from build123d import *

# Parameters (mm, degrees)
CROQUIS1_W              = 70
CROQUIS1_H              = 22
SALIENTE_EXTRUIR1_DEPTH = 18
CROQUIS2_R              = 2.5
SALIENTE_EXTRUIR2_DEPTH = 10
REDONDEO3_R             = 5
REDONDEO4_R             = 5


with BuildPart() as part:
    # Croquis1 → Saliente-Extruir1 (new body)
    with BuildSketch(Plane.XY):
        with Locations((35, 11)):
            Rectangle(CROQUIS1_W, CROQUIS1_H)
    extrude(amount=SALIENTE_EXTRUIR1_DEPTH)

    # Croquis2 → Saliente-Extruir2 (add)
    with BuildSketch(Plane.XY.offset(18)):
        with Locations(Location((59.5, 11, 0), (0, 0, 180))):
            Circle(CROQUIS2_R)
    extrude(amount=SALIENTE_EXTRUIR2_DEPTH)

    # Redondeo3
    redondeo3_edges = [part.edges().sort_by_distance(p)[0] for p in [
        (0, 22, 9),
    ]]
    fillet(redondeo3_edges, radius=REDONDEO3_R)

    # Redondeo4
    redondeo4_edges = [part.edges().sort_by_distance(p)[0] for p in [
        (0, 0, 9),
    ]]
    fillet(redondeo4_edges, radius=REDONDEO4_R)


solid = part.part
The model under review builds one solid part; all positions refer to its coordinate system, in mm. A direction names the side the tool comes from. Give positions to 0.01 mm unless a question says otherwise; leave off trailing zeros. Order: outer loops, then holes, each group sorted by start corner. A loop starts at its lowest first (then second) coordinate and runs counter-clockwise, first axis right, second up. Notation, with made-up numbers: (87, 46) -> (98, 46) arc R19 ccw to (98, 61) -> close; hole circle Ø11 at (47.5, 67.5). An arc over 180 degrees is marked (long way). Write item = value, one per line. Start each with the question number.
(1) Take a section at A-A (y = 11). Write out the cut boundary in (x, z).
(2) Take a section at B-B (x = 59.5). Write out the cut boundary in (y, z).
(3) For L1, parallel to Z at x = 28, y = 17; L2, parallel to X at y = 19.75, z = 6.5; L3, parallel to Y at x = 4, z = 8.75, list the stretches that pass through material, from the lowest coordinate up. Write a range as from..to.
(4) Tool access review of faces 1 (the flat face through (70, 11, 9)), 2 (the cylindrical face through (57.19, 11.96, 22.93)): name each direction out of +Z, -Z, +X, -X, +Y, -Y from which nothing blocks a thin tool from reaching the whole face with its end or side.
(5) For pin 1 Ø8 at (x, y) = (12, 12.5) entering from -Z, flat-tipped, find the tip position at first contact; note if it passes through.
(6) Take a section at D-D (y = 14.25). Write out the cut boundary in (x, z), plus the area to 3 significant figures.
(7) Take a section at C-C (z = 20.25). Write out the cut boundary in (x, y).
Returned:
q1.outline = (0, 0) -> (70, 0) -> (70, 18) -> (62, 18) -> (62, 28) -> (57, 28) -> (57, 18) -> (0, 18) -> close
q2.outline = (0, 0) -> (22, 0) -> (22, 18) -> (13.5, 18) -> (13.5, 28) -> (8.5, 28) -> (8.5, 18) -> (0, 18) -> close
q3.L1 = 0..18
q3.L2 = 0.82..70
q3.L3 = 0.1..21.9
q4.face_1 = +Z, -Z, +X, +Y, -Y
q4.face_2 = +Z
q5.pin_1 = 0
q6.outline = (0, 0) -> (70, 0) -> (70, 18) -> (0, 18) -> close
q6.area = 1,260 mm²
q7.outline = circle Ø5 at (59.5, 11)
